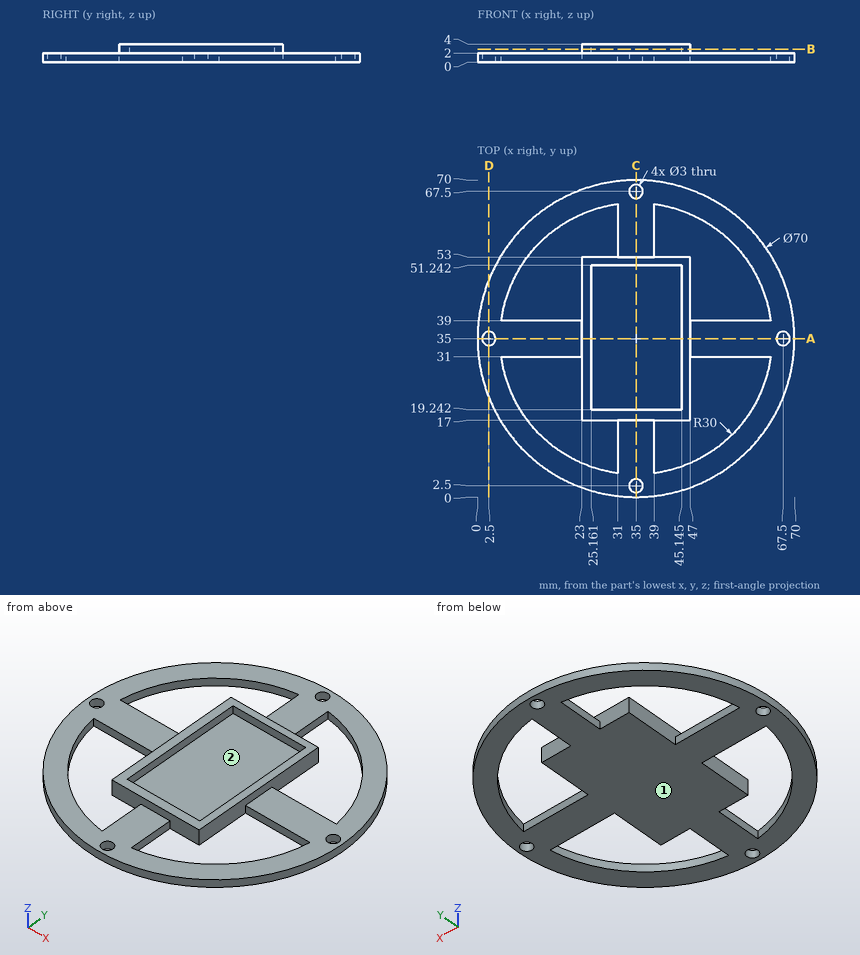
Could you check a few things on this drawing? It's one solid part, dimensions in mm from its lowest x, y, z. Coordinates: 2 decimals unless noted, no trailing zeros. Write each loop counter-clockwise with the first axis right and the second up, starting at its lowest first coordinate (ties: lowest second). Pieces come first, ordered by that corner, then holes.
Q1. If we mould it in two halves opening along X, with no side actions, what happens to the marked faces 1 and 2? For each: +X half, -X half, draft (parallel to the pull), parting line (faces both ways), or undercut.
Results found:
face 1: draft
face 2: undercut
Q2. Imagine slicing it at C-C, the plane x = 35. List the corners of the cut face in (y, z) for me.
Results found:
outline: (0, 0) - (1, 0) - (1, 2) - (0, 2) - close; (4, 0) - (66, 0) - (66, 2) - (53, 2) - (53, 4) - (51.24, 4) - (51.24, 2) - (19.24, 2) - (19.24, 4) - (17, 4) - (17, 2) - (4, 2) - close; (69, 0) - (70, 0) - (70, 2) - (69, 2) - close
Q3. Imagine slicing it at D-D, the plane x = 2.5. List the corners of the cut face in (y, z) for me.
Results found:
outline: (22.01, 0) - (33.5, 0) - (33.5, 2) - (22.01, 2) - close; (36.5, 0) - (47.99, 0) - (47.99, 2) - (36.5, 2) - close
Q4. Imagine slicing it at A-A, the plane y = 35. List the corners of the cut face in (x, z) for me (1 decimal).
Results found:
outline: (0, 0) - (1, 0) - (1, 2) - (0, 2) - close; (4, 0) - (66, 0) - (66, 2) - (47, 2) - (47, 4) - (45.1, 4) - (45.1, 2) - (25.2, 2) - (25.2, 4) - (23, 4) - (23, 2) - (4, 2) - close; (69, 0) - (70, 0) - (70, 2) - (69, 2) - close
Q5. Imagine slicing it at B-B, the plane z = 2.85. List the corners of the cut face in (x, y) for me (1 decimal).
Results found:
outline: (23, 17) - (47, 17) - (47, 53) - (23, 53) - close; hole (25.2, 19.2) - (45.1, 19.2) - (45.1, 51.2) - (25.2, 51.2) - close
Q6. For P1, Ø3.5, axis at x = 35, y = 2.5, coming from the +Z side; P2, Ø1.5, axis at y = 34, z = 2.5, coming from the +X side; P3, Ø2, axis at x = 38, z = 1.5, coming from the -Y side; P4, Ø1.8, axis at x = 67.5, y = 35, coming from the -Z side, each with a flat end and sliding along its axis, tell me the tip position at first contact or that it passes through.
Results found:
P1: stops at z = 2
P2: stops at x = 70
P3: stops at y = 0.06
P4: passes through
Q7. Please list where these lines run through material, in increasing order: L1, parallel to Y at x = 35, z = 1.3; L2, parallel to Y at x = 50, z = 0.5; L3, parallel to Y at x = 33.5, z = 3.15.
Results found:
L1: y = 0 to 1, 4 to 66, 69 to 70
L2: y = 3.38 to 9.02, 31 to 39, 60.98 to 66.62
L3: y = 17 to 19.24, 51.24 to 53
